Could you check a few things on this drawing? It's one solid part, dimensions in mm from its lowest x, y, z. A direction names the side the tool comes from. Round coordinates to 2 decimals unless told otherwise and drop trailing zeros. Loops run counter-clockwise (first coordinate to the right, second up) from the corner with the lowest first, then second, coordinate; pieces in that order, holes last. Notation, with made-up numbers: (76.5, 11) -> (133.5, 11) arc R20 ccw to (133.5, 46) -> close; hole circle Ø1 at (7.25, 87.25). An arc over 180 degrees is marked (long way). Put each result on its own line as item: value. Start each with the question number.
1. I need wall thicknesses on line 1 (Y direction, x = 9.25, z = 0.65); line 2 (Y direction, x = 10.75, z = 2); line 3 (X direction, y = 15, z = 2.5). Which ranges of each line are inside material? Lowest first, please. Write a range as [from, to].
2. Imagine slicing it at B-B, the plane z = 3. Please give me the cut outline in (x, y), and give its area (3 significant figures).
3. Imagine slicing it at C-C, the plane x = 9.25. Please give me the cut outline in (y, z), and give its area (3 significant figures).
4. Imagine slicing it at D-D, the plane z = 8.5. Please give me the cut outline in (x, y).
5. Which directions (+Z, -Z, +X, -X, +Y, -Y) give clear straight access to the entire face, cutting with the end or side of a thin tool? Please do the marked faces 1, 2, 3 and 4.
6. I'm going to push flat-ended pins straight in: P1, Ø5, axis at x = 10.5, y = 6, coming from the +Z side; P2, Ø2, axis at y = 11.5, z = 5.5, coming from the +X side; P3, Ø0.8, axis at x = 9.5, y = 0.5, coming from the +Z side; P4, Ø3, axis at x = 10.5, z = 7.5, coming from the +Y side. Where does each tip first touch, or does it pass through?
7. If we mould it in two halves opening along X, with no side actions, what happens to the marked faces 5, 6, 7 and 8? For each: pulls with the +X half, pulls with the -X half, needs draft (parallel to the pull), parting line crosses it, or undercut.
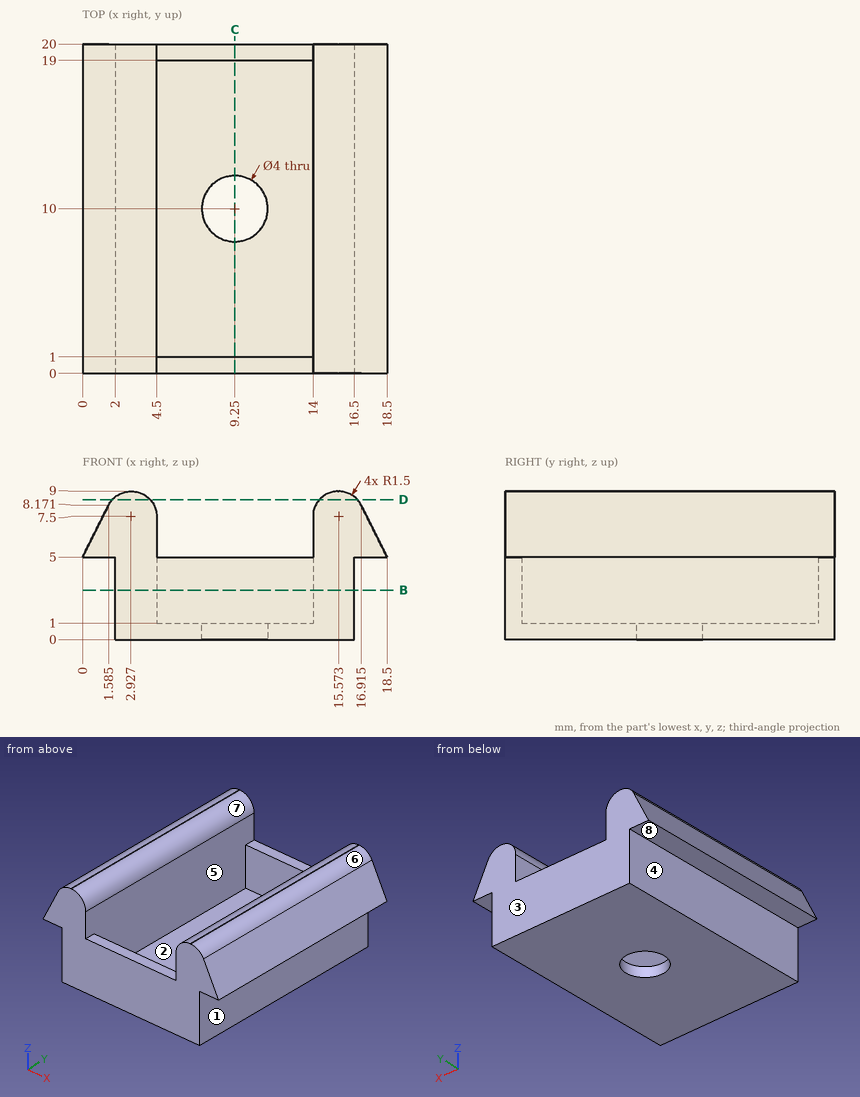
Entries:
1. line 1: [0, 8], [12, 20]
1. line 2: [0, 1], [19, 20]
1. line 3: [2, 4.5], [14, 16.5]
2. outline: (2, 0) -> (16.5, 0) -> (16.5, 20) -> (2, 20) -> close; hole (4.5, 1) -> (14, 1) -> (14, 19) -> (4.5, 19) -> close
2. area: 119 mm^2
3. outline: (0, 0) -> (8, 0) -> (8, 1) -> (1, 1) -> (1, 5) -> (0, 5) -> close; (12, 0) -> (20, 0) -> (20, 5) -> (19, 5) -> (19, 1) -> (12, 1) -> close
3. area: 24.0 mm^2
4. outline: (1.81, 0) -> (4.12, 0) -> (4.12, 20) -> (1.81, 20) -> close; (14.38, 0) -> (16.69, 0) -> (16.69, 20) -> (14.38, 20) -> close
5. face 1: -Z, +X, +Y, -Y
5. face 2: +Z
5. face 3: +Z, -Z, +X, -X, +Y
5. face 4: -Z, -X, +Y, -Y
6. P1: z = 1
6. P2: x = 18.5
6. P3: z = 5
6. P4: through
7. face 5: undercut
7. face 6: pulls with the +X half
7. face 7: undercut
7. face 8: needs draft
